Input: part model. Units: mm. Frame: model coordinates. A direction names the side the tool comes from. Coordinates: 2 decimals unless noted, no trailing zeros. Order: outer loops, then holes, each group sorted by start corner. A loop starts at its lowest first (then second) coordinate and runs counter-clockwise, first axis right, second up. Notation, with made-up numbers: (-4.5, 83) -> (22.5, 83) arc R21 cw to (22.5, 107) -> close; hole circle Ø8 at (3.5, 16.5). An arc over 180 degrees is marked (long way). One line per question, with ' | ' between items.
```python
from build123d import *

# Parameters (mm, degrees)
SKETCH1_W           = 500
SKETCH1_H           = 350
BOSS_EXTRUDE1_DEPTH = 100
SKETCH2_R           = 10
CUT_EXTRUDE1_DEPTH  = 619.465843843
REVOLVE1_ANGLE      = 180
SKETCH4_R           = 25
BOSS_EXTRUDE2_DEPTH = 80
SKETCH5_W           = 100
SKETCH5_H           = 350
BOSS_EXTRUDE3_DEPTH = 40


with BuildPart() as part:
    # Sketch1 → Boss-Extrude1 (new body)
    with BuildSketch(Plane.XY):
        with Locations((250, -175)):
            Rectangle(SKETCH1_W, SKETCH1_H)
    extrude(amount=BOSS_EXTRUDE1_DEPTH)

    # Sketch2 → Cut-Extrude1 (cut, through all)
    with BuildSketch(Plane.XZ.offset(350)):
        with Locations(Location((80, 40, 0), (0, 0, 270))):
            Circle(SKETCH2_R)
    extrude(amount=-CUT_EXTRUDE1_DEPTH, mode=Mode.SUBTRACT)

    # Sketch3 → Revolve1 (revolve)
    with BuildSketch(Plane(origin=(0, 0, 0), x_dir=(-1, 0, 0), z_dir=(0, 0, -1))):
        with BuildLine():
            Line((-440, -175), (-320, -175))
            ThreePointArc((-320, -175), (-380, -235), (-440, -175))
        make_face()
    revolve(axis=Axis((500, -175, 0), (1, 0, 0)), revolution_arc=REVOLVE1_ANGLE)

    # Sketch4 → Boss-Extrude2 (add)
    with BuildSketch(Plane(origin=(500, 0, 0), x_dir=(0, 0, -1), z_dir=(1, 0, 0))):
        with Locations(Location((-50, -175, 0), (0, 0, 270))):
            Circle(SKETCH4_R)
    extrude(amount=BOSS_EXTRUDE2_DEPTH)

    # Sketch5 → Boss-Extrude3 (add)
    with BuildSketch(Plane(origin=(580, 0, 0), x_dir=(0, 0, -1), z_dir=(1, 0, 0))):
        with Locations((-50, -175)):
            Rectangle(SKETCH5_W, SKETCH5_H)
    extrude(amount=BOSS_EXTRUDE3_DEPTH)


solid = part.part
```
1. Cut plane B-B, the plane x = 80. Return loops of the section in (y, z).
Recorded:
outline: (-350, 0) -> (0, 0) -> (0, 30) -> (-350, 30) -> close; (-350, 50) -> (0, 50) -> (0, 100) -> (-350, 100) -> close
2. Pin query (flat end, axial travel): pin 1 Ø6 at (x, y) = (483, -83) entering from -Z; pin 2 Ø16 at (x, z) = (80, 40) entering from -Y; pin 3 Ø2 at (y, z) = (-153, -40) entering from +X. Return the tip coordinate at first contact, or that it passes through.
Recorded:
pin 1: stops at z = 0 | pin 2: passes through | pin 3: stops at x = 420.08
3. Ray query, line 1 (X direction, y = -93, z = 0.5); line 2 (X direction, y = -226, z = 40); line 3 (Z direction, x = 333, y = -214). Return the intervals inside material, ascending. Write a range as [from, to].
Recorded:
line 1: x = [0, 500], [580, 620] | line 2: x = [0, 70], [90, 500], [580, 620] | line 3: z = [0, 100]
4. Mould query, pull axis Z, two halves, no side actions, for faces 4 (the face through (600, -177, 100)), 5 (the face through (89.915, -177.45, 41.302)), 6 (the face through (247, 0, 49)). Classes: released by +Z, released by -Z, zero draft, split by the parting line, or undercut.
Recorded:
face 4: released by +Z | face 5: undercut | face 6: zero draft
5. Cut plane C-C, the plane y = -175. Return loops of the section in (x, z).
Recorded:
outline: (0, 0) -> (320, 0) arc R60 ccw to (440, 0) -> (500, 0) -> (500, 25) -> (580, 25) -> (580, 0) -> (620, 0) -> (620, 100) -> (580, 100) -> (580, 75) -> (500, 75) -> (500, 100) -> (0, 100) -> close; hole circle Ø20 at (80, 40)
6. Access query for faces 1 (the face through (600, -177, 0)), 2 (the face through (539.44, -198.09, 59.58)), 3 (the face through (247, -350, 49)). Directions: +Z, -Z, +X, -X, +Y, -Y. A direction counts if a zero-diameter tool reaches every point of the face in a straight line with its end or side. Return the directions, or none.
Recorded:
face 1: -Z, +X, +Y, -Y | face 2: none | face 3: +Z, -Z, +X, -X, -Y
7. Cut plane D-D, the plane z = 40. Return loops of the section in (x, y), and give its area (3 significant figures).
Recorded:
outline: (0, -350) -> (70, -350) -> (70, 0) -> (0, 0) -> close; (90, -350) -> (500, -350) -> (500, -197.91) -> (580, -197.91) -> (580, -350) -> (620, -350) -> (620, 0) -> (580, 0) -> (580, -152.09) -> (500, -152.09) -> (500, 0) -> (90, 0) -> close | area: 186,000 mm^2
8. Cut plane A-A, the plane y = -249. Return loops of the section in (x, z), and give its area (3 significant figures).
Recorded:
outline: (0, 0) -> (500, 0) -> (500, 100) -> (0, 100) -> close; (580, 0) -> (620, 0) -> (620, 100) -> (580, 100) -> close; hole circle Ø20 at (80, 40) | area: 53,700 mm^2
